Read the model definition and answer for the solid it produces. Units are mm, in the model's axes. A direction names the side the tool comes from. Round coordinates to 2 decimals unless told otherwise and drop trailing zeros. Write each loop counter-clockwise with the first axis right and the second up, starting at its lowest first coordinate (ties: lowest second). Pieces come first, ordered by that corner, then holes.
from build123d import *

# Parameters (mm, degrees)
SKETCH1_R           = 18
SKETCH1_R_2         = 2
SKETCH1_W           = 10.25
SKETCH1_H           = 10.25
BOSS_EXTRUDE1_DEPTH = 27
CUT_EXTRUDE1_START  = -7
CUT_EXTRUDE1_DEPTH  = 7
SKETCH4_W           = 9.35
SKETCH4_H           = 9.35
CUT_EXTRUDE3_DEPTH  = 15.4
CUT_EXTRUDE4_START  = -40
CUT_EXTRUDE4_DEPTH  = 40
SKETCH6_R           = 1.5
CUT_EXTRUDE5_DEPTH  = 48
SKETCH7_R           = 3
CUT_EXTRUDE6_DEPTH  = 3
CUT_EXTRUDE7_DEPTH  = 4
CHAMFER1_SIZE       = 1
CHAMFER1_SIZE_2     = 2.747477419
CUT_EXTRUDE8_DEPTH  = 37.633318168
SKETCH12_R          = 1.4
CUT_EXTRUDE10_DEPTH = 20
CUT_EXTRUDE9_START  = -4
SKETCH10_R          = 18
SKETCH10_R_2        = 16
CUT_EXTRUDE9_DEPTH  = 4


with BuildPart() as part:
    # Sketch1 → Boss-Extrude1 (new body)
    with BuildSketch(Plane(origin=(0, 0, 0), x_dir=(1, 0, 0), z_dir=(0, 1, 0))):
        with Locations(Location((0, 0, 0), (0, 0, 270))):
            Circle(SKETCH1_R)
        with Locations(Location((-12, 0, 0), (0, 0, 270))):
            Circle(SKETCH1_R_2, mode=Mode.SUBTRACT)
        Rectangle(SKETCH1_W, SKETCH1_H, mode=Mode.SUBTRACT)
    extrude(amount=BOSS_EXTRUDE1_DEPTH)

    # Sketch2 → Cut-Extrude1 (cut)
    with BuildSketch(Plane(origin=(0, 27, 0), x_dir=(1, 0, 0), z_dir=(0, 1, 0)).offset(CUT_EXTRUDE1_START)):
        with BuildLine():
            Line((-10.8, 5), (-17.291616466, 5))
            ThreePointArc((-17.291616466, 5), (-18, 0), (-17.291616466, -5))
            Line((-17.291616466, -5), (-10.8, -5))
            ThreePointArc((-10.8, -5), (-5.8, 0), (-10.8, 5))
        make_face()
    extrude(amount=CUT_EXTRUDE1_DEPTH, mode=Mode.SUBTRACT)

    # Sketch4 → Cut-Extrude3 (cut)
    with BuildSketch(Plane(origin=(0, 0, 0), x_dir=(-1, 0, 0), z_dir=(0, -1, 0))):
        with Locations((11.135393506, 0.872889968)):
            Rectangle(SKETCH4_W, SKETCH4_H)
    extrude(amount=-CUT_EXTRUDE3_DEPTH, mode=Mode.SUBTRACT)

    # Sketch5 → Cut-Extrude4 (cut)
    with BuildSketch(Plane(origin=(0, 27, 0), x_dir=(1, 0, 0), z_dir=(0, 1, 0)).offset(CUT_EXTRUDE4_START)):
        with BuildLine():
            Line((5.916079783, 17), (-5.916079783, 17))
            ThreePointArc((-5.916079783, 17), (0, 18), (5.916079783, 17))
        make_face()
        with BuildLine():
            Line((5.916079783, -17), (-5.916079783, -17))
            ThreePointArc((-5.916079783, -17), (0, -18), (5.916079783, -17))
        make_face()
    extrude(amount=CUT_EXTRUDE4_DEPTH, mode=Mode.SUBTRACT)

    # Sketch6 → Cut-Extrude5 (cut, through all)
    with BuildSketch(Plane(origin=(0, 0, -17), x_dir=(-1, 0, 0), z_dir=(0, 0, -1))):
        with Locations((0, 17)):
            Circle(SKETCH6_R)
        with Locations((0, 5)):
            Circle(SKETCH6_R)
    extrude(amount=-CUT_EXTRUDE5_DEPTH, mode=Mode.SUBTRACT)

    # Sketch7 → Cut-Extrude6 (cut)
    with BuildSketch(Plane(origin=(0, 0, -17), x_dir=(-1, 0, 0), z_dir=(0, 0, -1))):
        with Locations((0, 17)):
            Circle(SKETCH7_R)
        with Locations((0, 5)):
            Circle(SKETCH7_R)
    extrude(amount=-CUT_EXTRUDE6_DEPTH, mode=Mode.SUBTRACT)

    # Sketch8 → Cut-Extrude7 (cut)
    with BuildSketch(Plane.XY.offset(17)):
        Polygon((0, 13.8), (2.771281292, 15.4), (2.771281292, 18.6), (0, 20.2), (-2.771281292, 18.6), (-2.771281292, 15.4), align=None)
        Polygon((0, 1.8), (2.771281292, 3.4), (2.771281292, 6.6), (0, 8.2), (-2.771281292, 6.6), (-2.771281292, 3.4), align=None)
    extrude(amount=-CUT_EXTRUDE7_DEPTH, mode=Mode.SUBTRACT)

    # Chamfer1
    # the kernel refuses this chamfer: 2.747477419, 1 mm, written as the material it takes off along each edge
    with BuildSketch(Plane(origin=(-5.125, 27, -5.125), x_dir=(0, 0.09904090225204956, -0.9950833631817488), z_dir=(1, 0, 0)), Plane(origin=(-5.125, 27, 5.125), x_dir=(-0.9950833631817488, 0.09904090225204956, 0), z_dir=(0, 0, -1)), Plane(origin=(5.125, 27, 5.125), x_dir=(0, 0.09904090225204956, 0.9950833631817488), z_dir=(-1, 0, 0)), Plane(origin=(5.125, 27, -5.125), x_dir=(0.9950833631817488, 0.09904090225204956, 0), z_dir=(0, 0, 1))) as chamfer1_piece_1:
        Polygon((CHAMFER1_SIZE * 0.995083363182, -CHAMFER1_SIZE * 0.099040902252), (-CHAMFER1_SIZE_2 * 0.0990409022684, -CHAMFER1_SIZE_2 * 0.995083363346), (0, 0), align=None)
    extrude(amount=10.25, mode=Mode.SUBTRACT)
    with BuildSketch(Plane(origin=(-5.125, 27, 5.125), x_dir=(-0.9950833631817488, 0.09904090225204956, 0), z_dir=(0, 0, -1))) as chamfer1_piece_2a_section:
        Polygon((CHAMFER1_SIZE * 0.995083363182, -CHAMFER1_SIZE * 0.099040902252), (-CHAMFER1_SIZE_2 * 0.0990409022684, -CHAMFER1_SIZE_2 * 0.995083363346), (0, 0), align=None)
    chamfer1_piece_2a = extrude(amount=17.377491449, mode=Mode.PRIVATE)
    chamfer1_piece_2a = split(chamfer1_piece_2a, bisect_by=Plane(origin=(-5.432505006, 26.059901151, -5.125), z_dir=(0, 0, -1)), keep=Keep.TOP, mode=Mode.PRIVATE)
    with BuildSketch(Plane(origin=(-12.252491449, 27, -5.125), x_dir=(0, 0.09904090225204956, -0.9950833631817488), z_dir=(1, 0, 0))) as chamfer1_piece_2b_section:
        Polygon((CHAMFER1_SIZE * 0.995083363182, -CHAMFER1_SIZE * 0.099040902252), (-CHAMFER1_SIZE_2 * 0.0990409022684, -CHAMFER1_SIZE_2 * 0.995083363346), (0, 0), align=None)
    chamfer1_piece_2b = extrude(amount=17.377491449, mode=Mode.PRIVATE)
    chamfer1_piece_2b = split(chamfer1_piece_2b, bisect_by=Plane(origin=(-5.125, 26.059901151, -5.432505006), z_dir=(-1, 0, 0)), keep=Keep.TOP, mode=Mode.PRIVATE)
    chamfer1_piece_2 = chamfer1_piece_2a & chamfer1_piece_2b
    add(chamfer1_piece_2, mode=Mode.SUBTRACT)
    with BuildSketch(Plane(origin=(5.125, 27, -12.252491449), x_dir=(0.9950833631817488, 0.09904090225204956, 0), z_dir=(0, 0, 1))) as chamfer1_piece_3a_section:
        Polygon((CHAMFER1_SIZE * 0.995083363182, -CHAMFER1_SIZE * 0.099040902252), (-CHAMFER1_SIZE_2 * 0.0990409022684, -CHAMFER1_SIZE_2 * 0.995083363346), (0, 0), align=None)
    chamfer1_piece_3a = extrude(amount=17.377491449, mode=Mode.PRIVATE)
    chamfer1_piece_3a = split(chamfer1_piece_3a, bisect_by=Plane(origin=(5.432505006, 26.059901151, -5.125), z_dir=(0, 0, -1)), keep=Keep.TOP, mode=Mode.PRIVATE)
    with BuildSketch(Plane(origin=(-5.125, 27, -5.125), x_dir=(0, 0.09904090225204956, -0.9950833631817488), z_dir=(1, 0, 0))) as chamfer1_piece_3b_section:
        Polygon((CHAMFER1_SIZE * 0.995083363182, -CHAMFER1_SIZE * 0.099040902252), (-CHAMFER1_SIZE_2 * 0.0990409022684, -CHAMFER1_SIZE_2 * 0.995083363346), (0, 0), align=None)
    chamfer1_piece_3b = extrude(amount=17.377491449, mode=Mode.PRIVATE)
    chamfer1_piece_3b = split(chamfer1_piece_3b, bisect_by=Plane(origin=(5.125, 26.059901151, -5.432505006), z_dir=(1, 0, 0)), keep=Keep.TOP, mode=Mode.PRIVATE)
    chamfer1_piece_3 = chamfer1_piece_3a & chamfer1_piece_3b
    add(chamfer1_piece_3, mode=Mode.SUBTRACT)
    with BuildSketch(Plane(origin=(5.125, 27, 5.125), x_dir=(0, 0.09904090225204956, 0.9950833631817488), z_dir=(-1, 0, 0))) as chamfer1_piece_4a_section:
        Polygon((CHAMFER1_SIZE * 0.995083363182, -CHAMFER1_SIZE * 0.099040902252), (-CHAMFER1_SIZE_2 * 0.0990409022684, -CHAMFER1_SIZE_2 * 0.995083363346), (0, 0), align=None)
    chamfer1_piece_4a = extrude(amount=17.377491449, mode=Mode.PRIVATE)
    chamfer1_piece_4a = split(chamfer1_piece_4a, bisect_by=Plane(origin=(-5.125, 26.059901151, 5.432505006), z_dir=(-1, 0, 0)), keep=Keep.TOP, mode=Mode.PRIVATE)
    with BuildSketch(Plane(origin=(-5.125, 27, 12.252491449), x_dir=(-0.9950833631817488, 0.09904090225204956, 0), z_dir=(0, 0, -1))) as chamfer1_piece_4b_section:
        Polygon((CHAMFER1_SIZE * 0.995083363182, -CHAMFER1_SIZE * 0.099040902252), (-CHAMFER1_SIZE_2 * 0.0990409022684, -CHAMFER1_SIZE_2 * 0.995083363346), (0, 0), align=None)
    chamfer1_piece_4b = extrude(amount=17.377491449, mode=Mode.PRIVATE)
    chamfer1_piece_4b = split(chamfer1_piece_4b, bisect_by=Plane(origin=(-5.432505006, 26.059901151, 5.125), z_dir=(0, 0, 1)), keep=Keep.TOP, mode=Mode.PRIVATE)
    chamfer1_piece_4 = chamfer1_piece_4a & chamfer1_piece_4b
    add(chamfer1_piece_4, mode=Mode.SUBTRACT)
    with BuildSketch(Plane(origin=(12.252491449, 27, 5.125), x_dir=(0, 0.09904090225204956, 0.9950833631817488), z_dir=(-1, 0, 0))) as chamfer1_piece_5a_section:
        Polygon((CHAMFER1_SIZE * 0.995083363182, -CHAMFER1_SIZE * 0.099040902252), (-CHAMFER1_SIZE_2 * 0.0990409022684, -CHAMFER1_SIZE_2 * 0.995083363346), (0, 0), align=None)
    chamfer1_piece_5a = extrude(amount=17.377491449, mode=Mode.PRIVATE)
    chamfer1_piece_5a = split(chamfer1_piece_5a, bisect_by=Plane(origin=(5.125, 26.059901151, 5.432505006), z_dir=(1, 0, 0)), keep=Keep.TOP, mode=Mode.PRIVATE)
    with BuildSketch(Plane(origin=(5.125, 27, -5.125), x_dir=(0.9950833631817488, 0.09904090225204956, 0), z_dir=(0, 0, 1))) as chamfer1_piece_5b_section:
        Polygon((CHAMFER1_SIZE * 0.995083363182, -CHAMFER1_SIZE * 0.099040902252), (-CHAMFER1_SIZE_2 * 0.0990409022684, -CHAMFER1_SIZE_2 * 0.995083363346), (0, 0), align=None)
    chamfer1_piece_5b = extrude(amount=17.377491449, mode=Mode.PRIVATE)
    chamfer1_piece_5b = split(chamfer1_piece_5b, bisect_by=Plane(origin=(5.432505006, 26.059901151, 5.125), z_dir=(0, 0, 1)), keep=Keep.TOP, mode=Mode.PRIVATE)
    chamfer1_piece_5 = chamfer1_piece_5a & chamfer1_piece_5b
    add(chamfer1_piece_5, mode=Mode.SUBTRACT)

    # Sketch9 → Cut-Extrude8 (cut, through all)
    with BuildSketch(Plane.XZ):
        with BuildLine():
            Line((-7.454203172, -7.297889968), (-15.454203172, -7.297889968))
            ThreePointArc((-15.454203172, -7.297889968), (-13.761984914, -9.955415688), (-11.632322635, -12.277178848))
            Line((-11.632322635, -12.277178848), (-7.454203172, -7.297889968))
        make_face()
    extrude(amount=-CUT_EXTRUDE8_DEPTH, mode=Mode.SUBTRACT)

    # Sketch12 → Cut-Extrude10 (cut)
    with BuildSketch(Plane(origin=(0, 27, 0), x_dir=(1, 0, 0), z_dir=(0, 1, 0))):
        with Locations(Location((10, 0, 0), (0, 0, 270))):
            Circle(SKETCH12_R)
        with Locations(Location((-9.192388155, -9.192388155, 0), (0, 0, 270))):
            Circle(SKETCH12_R)
    extrude(amount=-CUT_EXTRUDE10_DEPTH, mode=Mode.SUBTRACT)

    # Sketch10 → Cut-Extrude9 (cut)
    with BuildSketch(Plane(origin=(0, 27, 0), x_dir=(1, 0, 0), z_dir=(0, 1, 0)).offset(CUT_EXTRUDE9_START)):
        Circle(SKETCH10_R)
        Circle(SKETCH10_R_2, mode=Mode.SUBTRACT)
    extrude(amount=CUT_EXTRUDE9_DEPTH, mode=Mode.SUBTRACT)


solid = part.part
Q1. Straight lines are drawn through the part: probe 1 along X at (y, z) = (18, 0) (3 decimals); probe 2 along Y at (x, z) = (0, 7.25); probe 3 along Y at (x, z) = (-1, 15.5). For each, find the intervals that lie inside material, in ascending order.
Verdict:
probe 1: x = -18 to -14, -10 to -5.125, 5.125 to 8.6, 11.4 to 18
probe 2: y = 0 to 3.5, 6.5 to 15.5, 18.5 to 27
probe 3: y = 0 to 2.38, 7.62 to 14.38, 19.62 to 27
Q2. Flat-ended cylindrical pins translate along their axes: pin 1 Ø2 at (y, z) = (8, 8.5) entering from -X; pin 2 Ø1.7 at (x, y) = (1, 4.5) entering from +Z; pin 3 Ø2.5 at (x, y) = (0, 17) entering from -Z; pin 4 Ø4.5 at (x, z) = (-11.5, -2.5) entering from -Y. Find the tip coordinate at first contact, or state that the pin passes through.
Verdict:
pin 1: stops at x = -16.36
pin 2: stops at z = 13
pin 3: passes through
pin 4: stops at y = 15.4
Q3. Section A-A (y = 17) is taken. State how many separate pieces and enclosed holes the cut face has, then the cut area to 3 significant figures.
Verdict:
separate pieces: 2
enclosed holes: 4
area: 761 mm2
Q4. Section D-D (x = 10) is taken. Determine the outline of the cut face in (y, z).
Verdict:
outline: (0, -14.97) - (23, -14.97) - (23, -12.49) - (27, -12.49) - (27, -1.4) - (7, -1.4) - (7, 1.4) - (27, 1.4) - (27, 12.49) - (23, 12.49) - (23, 14.97) - (0, 14.97) - close
Q5. Which of the six approach directions +Z, -Z, +X, -X, +Y, -Y give full straight-line access (tool end or side, diameter ignored) to faces 4 (the flat face through (-11, 8, -5.548)), 5 (the flat face through (-5.125, 12, 0)), 6 (the flat face through (16, 23, 2.4)), 7 (the flat face through (-1.3, 15.6, 13))?
Verdict:
face 4: -Y
face 5: +Y, -Y
face 6: +Y
face 7: +Z
Q6. Section B-B (z = -13) is taken. Determine the outline of the cut face in (x, y).
Verdict:
outline: (-12.45, 0) - (12.45, 0) - (12.45, 23) - (9.33, 23) - (9.33, 27) - (-9.33, 27) - (-9.33, 23) - (-12.45, 23) - close; hole circle Ø3 at (0, 5); hole circle Ø3 at (0, 17)
Q7. Section C-C (y = 23.75) is taken. Determine the outline of the cut face in (x, z) (1 decimal).
Verdict:
outline: (-15.2, -5) arc R16 ccw to (-14.2, -7.3) - (-7.5, -7.3) - (-11, -11.6) arc R16 ccw (long way) to (-15.2, 5) - (-10.8, 5) arc R5 cw to (-10.8, -5) - close; hole circle Ø2.8 at (-9.2, 9.2); hole (-5.1, -5.1) - (5.1, -5.1) - (5.1, 5.1) - (-5.1, 5.1) - close; hole circle Ø2.8 at (10, 0)
Q8. Determine the mould class of faces 1 (the flat face through (-0.086, 25.645, -5.632)), 2 (the flat face through (-13, 23, 5)), 3 (the cylindrical face through (-14.76, 24.97, -6.18)) for opening direction X: pulls with the +X half, pulls with the -X half, needs draft (parallel to the pull), parting line crosses it, or undercut.
Verdict:
face 1: undercut
face 2: needs draft
face 3: pulls with the -X half
